Work out the finished part from the listing and answer in its coordinate system (mm). A direction names the side the tool comes from. Round coordinates to 2 decimals unless told otherwise and drop trailing zeros. Loops run counter-clockwise (first coordinate to the right, second up) from the corner with the lowest first, then second, coordinate; pieces in that order, holes last. Notation, with made-up numbers: (6.5, 76) -> (15.5, 76) arc R15 cw to (15.5, 97) -> close; hole circle Ø7 at (67, 60). An arc over 180 degrees is marked (long way). Use one line per item in the form item = value.
```python
from build123d import *

# Parameters (mm, degrees)
SKETCH1_R           = 1.5
BOSS_EXTRUDE1_DEPTH = 12.7
SKETCH3_R           = 2.25
BOSS_EXTRUDE2_DEPTH = 2
FILLET2_R           = 0.25
FILLET3_R           = 0.25


with BuildPart() as part:
    # Sketch1 → Boss-Extrude1 (new body)
    with BuildSketch(Plane.XY):
        Circle(SKETCH1_R)
    extrude(amount=BOSS_EXTRUDE1_DEPTH)

    # Sketch3 → Boss-Extrude2 (add)
    with BuildSketch(Plane.XY):
        Circle(SKETCH3_R)
    extrude(amount=-BOSS_EXTRUDE2_DEPTH)

    # Fillet2
    fillet2_edges = [part.edges().sort_by_distance(p)[0] for p in [
        (-1.5, 0, 12.7),
    ]]
    fillet(fillet2_edges, radius=FILLET2_R)

    # Fillet3
    fillet3_edges = [part.edges().sort_by_distance(p)[0] for p in [
        (-1.5, 0, 0),
    ]]
    fillet(fillet3_edges, radius=FILLET3_R)


solid = part.part
```
(1) Find section A-A, the plane x = 0. Write down the section's boundary in (y, z).
Completed:
outline = (-2.25, -2) -> (2.25, -2) -> (2.25, 0) -> (1.75, 0) arc R0.25 cw to (1.5, 0.25) -> (1.5, 12.45) arc R0.25 ccw to (1.25, 12.7) -> (-1.25, 12.7) arc R0.25 ccw to (-1.5, 12.45) -> (-1.5, 0.25) arc R0.25 cw to (-1.75, 0) -> (-2.25, 0) -> close
(2) Given P1, Ø1.5, axis at y = -0.5, z = 0, coming from the +X side; P2, Ø2, axis at x = 1.5, z = 6.5, coming from the +Y side, each flat-ended and moving along its own axis, determine where each tip first touches the part or whether it passes through.
Completed:
P1 = 2.25
P2 = 1.41
(3) Find section C-C, the plane z = 5.5. Write down the section's boundary in (x, y).
Completed:
outline = circle Ø3 at (0, 0)
(4) Find section D-D, the plane x = -1.9. Write down the section's boundary in (y, z).
Completed:
outline = (-1.21, -2) -> (1.21, -2) -> (1.21, 0) -> (-1.21, 0) -> close
(5) Consider L1, parallel to Z at x = -1.6, y = -0.85; L2, parallel to X at y = 1.45, z = -0.75; L3, parallel to Y at x = -0.2, z = -1. Determine where each line is inside the solid, lowest interval first.
Completed:
L1 = -2 to 0
L2 = -1.72 to 1.72
L3 = -2.24 to 2.24
(6) For faces 1 (the cylindrical face through (-0.29, 2.23, -0.99)), 2 (the cylindrical face through (-1.5, 0.07, 6.26)), determine the directions among +Z, -Z, +X, -X, +Y, -Y from which every point of the face is accessible in a straight line to the end or side of a thin tool.
Completed:
face_1 = +Z, -Z
face_2 = +Z
